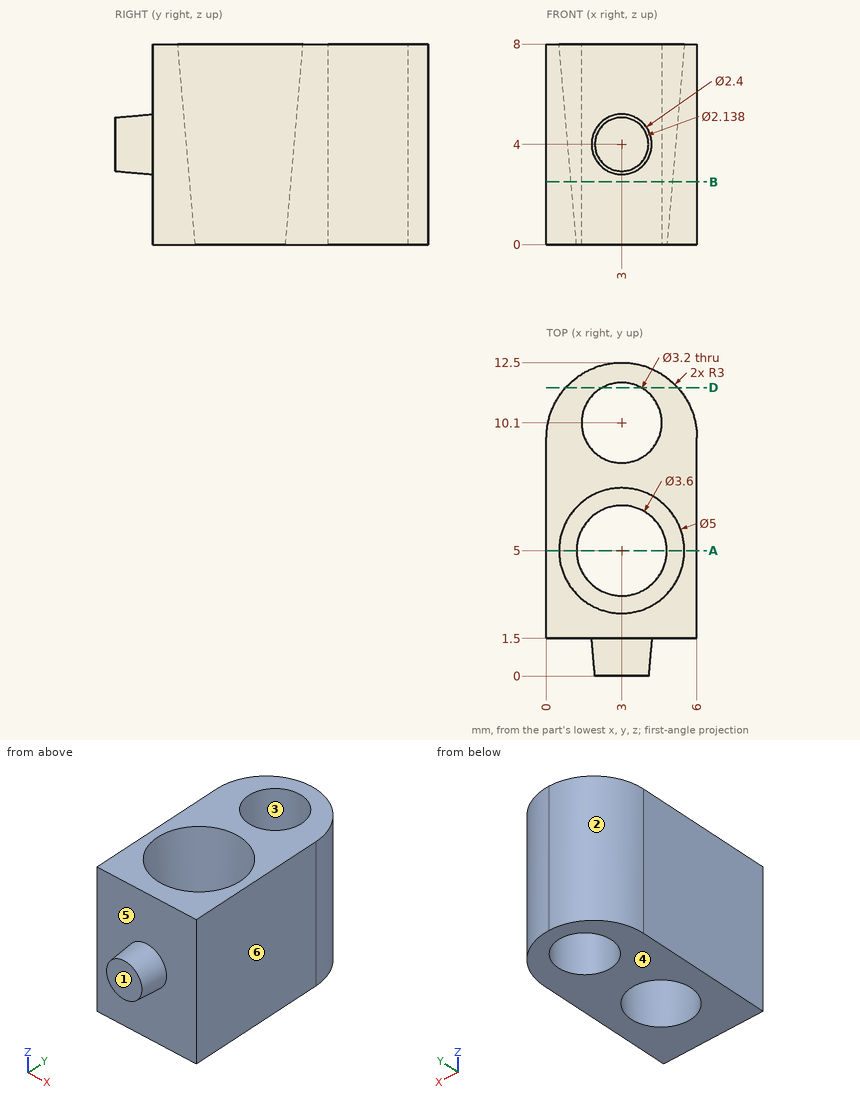
Job drawing, mm, ordinate dimensions from the low corner. One solid piece. A direction names the side the tool comes from. Give positions to 0.01 mm unless a question says otherwise; leave off trailing zeros. Write each loop counter-clockwise with the first axis right and the second up, starting at its lowest first coordinate (ties: lowest second). Pieces come first, ordered by that corner, then holes. Notation, with made-up numbers: M 3,88.25 L 30,88.25 A22 ccw 30,123.25 Z; hole C 11,34 d8. An arc over 180 degrees is marked long. One line per item, written item: value. Start each with the question number.
Q1. Saw through at B-B, the plane z = 2.5. State how many separate pieces and enclosed holes the cut face has.
Q2. 3-axis set-ups, long thin cutter, end or side, ignore diameter. For the marked faces 5 and 6: which of +Z, -Z, +X, -X, +Y, -Y reach the whole face in a straight line?
Q3. Saw through at D-D, the plane y = 11.5. Write the cut outline in (x, z) (1 decimal).
Q4. Probe probe 1 along Y at (x, z) = (3, 5.75); probe 2 along Y at (x, z) = (3, 4.25); probe 3 along X at (y, z) = (9, 7.5). List the from-to ranges inside material, lowest first. Write a range as [from, to].
Q5. Saw through at A-A, the plane y = 5. Write the cut outline in (x, z), plus the area to 3 significant figures.
Q6. Drop flat-ended pins along their axis: pin 1 Ø1.5 at (x, z) = (1, 4.5) entering from +Y; pin 2 Ø1.9 at (x, y) = (3, 10.1) entering from +Z (3 decimals). Give the stop position or say it passes through.
Q7. Two-plate mould, pull along Y, no slides. Class the marked faces 1, 2, 3 and 4: +Y half, -Y half, draft (parallel to the pull), parting line (faces both ways), or undercut.
Output values:
1. separate pieces: 1
1. enclosed holes: 2
2. face 5: -Y
2. face 6: +Z, -Z, +X, +Y, -Y
3. outline: M 0.8,0 L 2.2,0 L 2.2,8 L 0.8,8 Z; M 3.8,0 L 5.2,0 L 5.2,8 L 3.8,8 Z
4. probe 1: y = [1.5, 2.7], [7.3, 8.5], [11.7, 12.5]
4. probe 2: y = [0, 2.83], [7.17, 8.5], [11.7, 12.5]
4. probe 3: x = [0, 1.84], [4.16, 6]
5. outline: M 0,0 L 1.2,0 L 0.5,8 L 0,8 Z; M 4.8,0 L 6,0 L 6,8 L 5.5,8 Z
5. area: 13.6 mm²
6. pin 1: stops at y = 12.23
6. pin 2: passes through
7. face 1: -Y half
7. face 2: +Y half
7. face 3: undercut
7. face 4: draft
